The listing builds one solid part. Answer for the finished solid, in the listing's coordinates (mm). A direction names the side the tool comes from. Coordinates: 2 decimals unless noted, no trailing zeros. Write each loop counter-clockwise with the first axis right and the second up, starting at its lowest first coordinate (ties: lowest second). Pieces come first, ordered by that corner, then holes.
from build123d import *

# Parameters (mm, degrees)
F0_R     = 20
F1_DEPTH = 14
F2_R     = 20
F3_DEPTH = 20


with BuildPart() as f1:
    # F0 (on Front) → F1 (new body)
    with BuildSketch(Plane.XZ):
        Circle(F0_R)
        with BuildLine():
            ThreePointArc((-10.11945, -7.166362), (-12.4, 0), (-10.11945, 7.166362))
            ThreePointArc((-10.11945, 7.166362), (-9.682052, 10.512106), (-6.835723, 8.7))
            Line((-6.835723, 8.7), (6.835723, 8.7))
            ThreePointArc((6.835723, 8.7), (9.682052, 10.512106), (10.11945, 7.166362))
            ThreePointArc((10.11945, 7.166362), (12.4, 0), (10.11945, -7.166362))
            ThreePointArc((10.11945, -7.166362), (9.682052, -10.512106), (6.835723, -8.7))
            Line((6.835723, -8.7), (-6.835723, -8.7))
            ThreePointArc((-6.835723, -8.7), (-9.682052, -10.512106), (-10.11945, -7.166362))
        make_face(mode=Mode.SUBTRACT)
    extrude(amount=F1_DEPTH)

    # F2 (on face) → F3 (join)
    with BuildSketch(Plane.XZ.offset(14)):
        Circle(F2_R)
        with BuildLine():
            ThreePointArc((-6.45, 4.95), (-7.51066, 7.51066), (-4.95, 6.45))
            Line((-4.95, 6.45), (4.95, 6.45))
            ThreePointArc((4.95, 6.45), (7.51066, 7.51066), (6.45, 4.95))
            Line((6.45, 4.95), (6.45, -4.95))
            ThreePointArc((6.45, -4.95), (7.51066, -7.51066), (4.95, -6.45))
            Line((4.95, -6.45), (-4.95, -6.45))
            ThreePointArc((-4.95, -6.45), (-7.51066, -7.51066), (-6.45, -4.95))
            Line((-6.45, -4.95), (-6.45, 4.95))
        make_face(mode=Mode.SUBTRACT)
    extrude(amount=F3_DEPTH)


solid = f1.part
1. For a pull along X with two mould halves and no side action, classify faces 1 (the cylindrical face through (-4.336, -16.762, -19.524)), 2 (the cylindrical face through (7.475, -23.86, 7.545)), 3 (the flat face through (0, 0, 9)) as pulls with the +X half, pulls with the -X half, needs draft (parallel to the pull), parting line crosses it, or undercut.
Results found:
face 1: parting line crosses it
face 2: undercut
face 3: needs draft
2. Section B-B on x = 0 is taken. Give the vertices of the cut face in (y, z).
Results found:
outline: (-34, -20) - (0, -20) - (0, -8.7) - (-14, -8.7) - (-14, -6.45) - (-34, -6.45) - close; (-34, 6.45) - (-14, 6.45) - (-14, 8.7) - (0, 8.7) - (0, 20) - (-34, 20) - close
3. Section A-A on y = -26 is taken. Give the vertices of the cut face in (x, z), then the cut area to 3 significant figures.
Results found:
outline: circle Ø40 at (0, 0); hole (-6.45, -4.95) arc R1.5 ccw (long way) to (-4.95, -6.45) - (4.95, -6.45) arc R1.5 ccw (long way) to (6.45, -4.95) - (6.45, 4.95) arc R1.5 ccw (long way) to (4.95, 6.45) - (-4.95, 6.45) arc R1.5 ccw (long way) to (-6.45, 4.95) - close
area: 1,070 mm2
4. A tool of negligible diameter and unlimited length cuts with its end or side. For faces 4 (the cylindrical face through (-9.631, -6.902, -10.535)), 5 (the flat face through (0, -24, 6.45)), 6 (the flat face through (0, -34, -9)), from which of +Z, -Z, +X, -X, +Y, -Y can it reach the whole face along a straight path? Write none if from no direction.
Results found:
face 4: +Y
face 5: +Y, -Y
face 6: +Z, -Z, +X, -X, -Y
5. Find the intervals of material crossed by L1, parallel to X at y = -13, z = -0.5; L2, parallel to Z at x = 6.5, y = -24; L3, parallel to Y at x = 9, z = -9, in increasing order.
Results found:
L1: x = -19.99 to -12.39, 12.39 to 19.99
L2: z = -18.91 to -7.95, -4.95 to 4.95, 7.95 to 18.91
L3: y = -34 to -14
6. Section C-C on z = -3 is taken. Give the vertices of the cut face in (x, y), then the cut area to 3 significant figures.
Results found:
outline: (-19.77, -34) - (-6.45, -34) - (-6.45, -14) - (-12.03, -14) - (-12.03, 0) - (-19.77, 0) - close; (6.45, -34) - (19.77, -34) - (19.77, 0) - (12.03, 0) - (12.03, -14) - (6.45, -14) - close
area: 750 mm2
7. Flat-ended cylindrical pins translate along their axes: P1, Ø3, axis at x = 8.84, z = -8.7, coming from the +Y side; P2, Ø6.5, axis at x = 8.84, z = 8.7, coming from the +Y side; P3, Ø7, axis at x = 1, y = -5.5, coming from the -Z side; P4, Ø5, axis at x = -4.5, y = -5.5, coming from the -Z side. Find the tip coordinate at first contact, or state that the pin passes through.
Results found:
P1: stops at y = -14
P2: stops at y = 0
P3: stops at z = -20
P4: stops at z = -19.9
8. Section D-D on z = -10 is taken. Give the vertices of the cut face in (x, y), then the cut area to 3 significant figures.
Results found:
outline: (-17.32, -34) - (17.32, -34) - (17.32, 0) - (10.36, 0) - (10.36, -14) - (7.32, -14) - (7.32, 0) - (-7.32, 0) - (-7.32, -14) - (-10.36, -14) - (-10.36, 0) - (-17.32, 0) - close
area: 1,090 mm2
